Answer from the drawing. Dimensions are ordinates in mm from the lowest x, y and z of the part. A direction names the side the tool comes from. Coordinates: 2 decimals unless noted, no trailing zeros. Order: outer loops, then holes, each group sorted by start corner. A loop starts at its lowest first (then second) coordinate and runs counter-clockwise, first axis right, second up. Notation, with made-up numbers: (-32.75, -8.5) - (-19.75, -8.5) arc R33 cw to (-19.75, 19.5) - close; hole circle Ø4 at (16.5, 19.5). An arc over 180 degrees is marked (long way). Answer as a JSON object with one key per item and string values. Group by question number.
1) Section A-A (x = 151) is taken. Give the vertices of the cut face in (y, z), plus the area to 3 significant figures.
2) The mould has two halves that part along Y. Classify the marked faces 3, 4, 5 and 6: released by +Y, released by -Y, zero draft, split by the parting line, or undercut.
3) A tool of negligible diameter and unlimited length cuts with its end or side. For the marked faces 1 and 2, from which of +Z, -Z, +X, -X, +Y, -Y can it reach the whole face along a straight path? Write none if from no direction.
4) Section B-B (y = 67.5) is taken. Give the vertices of the cut face in (x, z), plus the area to 3 significant figures.
5) Section D-D (z = 13) is taken. Give the vertices of the cut face in (x, y), plus the area to 3 significant figures.
6) Section C-C (z = 27) is taken. Give the vertices of the cut face in (x, y).
7) Find the intervals of material crossed by line 1 along Y through (x, z) = (44, 43); line 2 along Y through (x, z) = (117, 17.5); line 3 along X through (y, z) = (28, 21), in increasing order.
8) Each of these flat-tipped pins is pushed along its axis until it touches: P1, Ø6, axis at y = 18, z = 13, coming from the +X side; P2, Ø3, axis at x = 50.5, y = 27.5, coming from the -Z side; P3, Ø6, axis at y = 37.5, z = 33.5, coming from the +X side. Where does it stop, or does it pass through?
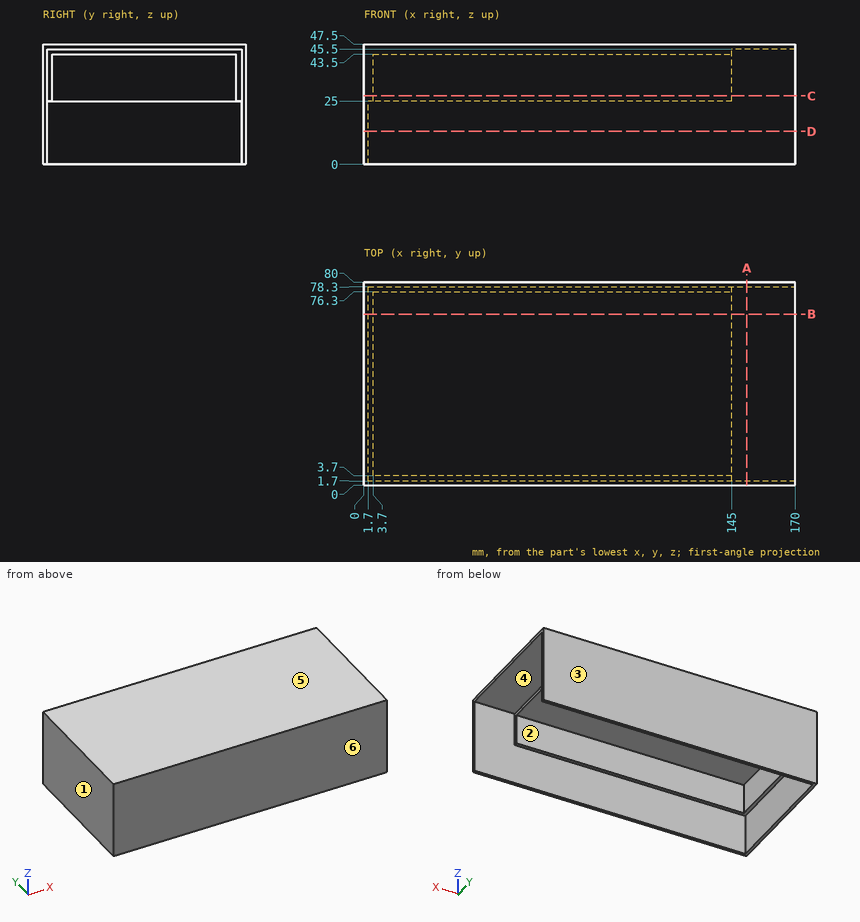
Report:
{
 "1": {"outline": "(0, 0) - (1.7, 0) - (1.7, 45.5) - (78.3, 45.5) - (78.3, 0) - (80, 0) - (80, 47.5) - (0, 47.5) - close", "area": "315 mm²"},
 "2": {"face 3": "released by +Y", "face 4": "undercut", "face 5": "zero draft", "face 6": "released by -Y"},
 "3": {"face 1": "+Z, -Z, -X, +Y, -Y", "face 2": "-Z, +X"},
 "4": {"outline": "(0, 0) - (1.7, 0) - (1.7, 25) - (3.7, 25) - (3.7, 43.5) - (145, 43.5) - (145, 45.5) - (170, 45.5) - (170, 47.5) - (0, 47.5) - close", "area": "741 mm²"},
 "5": {"outline": "(0, 0) - (170, 0) - (170, 1.7) - (1.7, 1.7) - (1.7, 78.3) - (170, 78.3) - (170, 80) - (0, 80) - close", "area": "708 mm²"},
 "6": {"outline": "(0, 0) - (170, 0) - (170, 1.7) - (145, 1.7) - (145, 3.7) - (3.7, 3.7) - (3.7, 76.3) - (145, 76.3) - (145, 78.3) - (170, 78.3) - (170, 80) - (0, 80) - close"},
 "7": {"line 1": "y = 0 to 3.7, 76.3 to 80", "line 2": "y = 0 to 1.7, 78.3 to 80", "line 3": "x = 0 to 1.7"},
 "8": {"P1": "stops at x = 1.7", "P2": "stops at z = 43.5", "P3": "stops at x = 3.7"}
}
